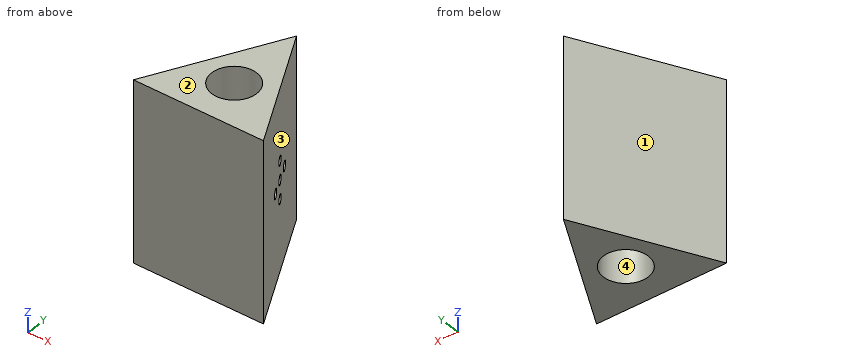
Autodesk Inventor part; units mm, degrees
ref_plane "YZ Plane" through (0, 0, 0) normal (1, 0, 0) x (0, 1, 0)
ref_plane "XZ Plane" through (0, 0, 0) normal (0, 1, 0) x (-1, 0, 0)
ref_plane "XY Plane" through (0, 0, 0) normal (0, 0, 1) x (1, 0, 0)
sketch "Sketch1" plane through (0, 0, 0) normal (0, 0, 1) x (1, 0, 0)
  circle A0 centre (0, 0) radius 4.7625
  line L0 (0, 0) -> (-0.0721, 14.2871)
  circle A1 centre (0, 0) radius 16.8508
  line L1 (-13.7645, -9.7205) -> (13.862, -9.581)
  line L2 (-13.7645, -9.7205) -> (-0.0851, 16.8506)
  line L3 (13.862, -9.581) -> (-0.0851, 16.8506)
  dimension "d0" = 9.525
extrude "Extrusion1" add sketch "Sketch1" along normal blind 38.1 contours L3 L1 L2
sketch "Sketch2" plane through (-0.0851, 16.8506, 38.1) normal (0.8844, 0.4667, 0) x (0, 0, -1)
  circle A0 centre (19.05, -14.9428) radius 1
  circle A1 centre (19.05, -10.9428) radius 1
  circle A2 centre (19.05, -18.9428) radius 1
  circle A3 centre (23.05, -14.9428) radius 1
  circle A4 centre (15.05, -14.9428) radius 1
  point P0 (38.1, -14.9428)
  dimension "d6" = 2
  dimension "d8" = 2
  dimension "d10" = 2
  dimension "d12" = 2
  dimension "d14" = 2
extrude "Extrusion2" cut sketch "Sketch2" against normal blind 2
sketch "Sketch3" plane through (0, 0, 38.1) normal (0, 0, 1) x (1, 0, 0)
  circle A0 centre (0, 0) radius 4.7625
  line L0 (-13.7645, -9.7205) -> (13.862, -9.581)
  line L1 (13.862, -9.581) -> (-0.0851, 16.8506)
  line L2 (-0.0851, 16.8506) -> (-13.7645, -9.7205)
properties part number "Triangle"
Here's how the part is built. I have some questions about the finished solid (model axes, mm). Face numbers are marked on the shaded views. Round coordinates to 2 decimals unless told otherwise and drop trailing zeros. Order: outer loops, then holes, each group sorted by start corner. A loop starts at its lowest first (then second) coordinate and runs counter-clockwise, first axis right, second up. Notation, with made-up numbers: M -23.75,-37 L 8.25,-37 A19 cw 8.25,-28 Z; hole C 45.25,-14 d3. An arc over 180 degrees is marked long. Answer in a Markdown table with one row per item.
Item 1: If I drill on L1, parallel to X at y = -0.25, z = 30; L2, parallel to Y at x = -4.25, z = 24; L3, parallel to X at y = -2, z = 36.5, over which ranges is the centre line in solid material (lowest first)? Write a range as from..to.
A:
| item | result |
|---|---|
| L1 | x = -8.89..-4.76, 4.76..8.94 |
| L2 | y = -9.67..-2.15, 2.15..8.76 |
| L3 | x = -9.79..-4.32, 4.32..9.86 |
Item 2: Imagine slicing it at C-C, the plane x = 1.5. Write out the boundary of the cut face in (y, z).
A:
| item | result |
|---|---|
| outline | M -9.64,0 L -4.52,0 L -4.52,38.1 L -9.64,38.1 Z; M 4.52,0 L 13.85,0 L 13.85,38.1 L 4.52,38.1 Z |
Item 3: I'm going to push flat-ended pins straight in: pin 1 (5 mm diameter, centred on x = 7, z = 9, fed in from -Y); pin 2 (3 mm diameter, centred on x = -7, z = 23.5, fed in from +Y); pin 3 (3 mm diameter, centred on y = 4, z = 27.5, fed in from +X). Where does each tip first touch, or does it pass through?
A:
| item | result |
|---|---|
| pin 1 | stops at y = -9.63 |
| pin 2 | stops at y = 6.33 |
| pin 3 | stops at x = 7.49 |
Item 4: Imagine slicing it at B-B, the plane z = 14.5. Write out the boundary of the cut face in (x, y) (1 decimal), and give its area (3 significant figures).
A:
| item | result |
|---|---|
| outline | M -13.8,-9.7 L 13.9,-9.6 L 7.3,2.9 L 5.5,2 L 4.7,3.4 L 6.5,4.4 L -0.1,16.9 Z; hole C 0,0 d9.5 |
| area | 291 mm2 |
Item 5: Imagine slicing it at A-A, the plane x = -3. Write out the boundary of the cut face in (y, z).
A:
| item | result |
|---|---|
| outline | M -9.67,0 L -3.7,0 L -3.7,38.1 L -9.67,38.1 Z; M 3.7,0 L 11.19,0 L 11.19,38.1 L 3.7,38.1 Z |
Item 6: Imagine slicing it at D-D, the plane z = 26.5. Write out the boundary of the cut face in (x, y) (1 decimal).
A:
| item | result |
|---|---|
| outline | M -13.8,-9.7 L 13.9,-9.6 L -0.1,16.9 Z; hole C 0,0 d9.5 |
Item 7: Thinking about a two-plate mould opening in X: for the marked faces 1, 2, 3 and 4, which applies, +X half, -X half, draft (parallel to the pull), parting line (faces both ways), or undercut?
A:
| item | result |
|---|---|
| face 1 | -X half |
| face 2 | draft |
| face 3 | +X half |
| face 4 | undercut |
